Autodesk Inventor part; units mm, degrees
ref_plane "YZ Plane" through (0, 0, 0) normal (1, 0, 0) x (0, 1, 0)
ref_plane "XZ Plane" through (0, 0, 0) normal (0, 1, 0) x (-1, 0, 0)
ref_plane "XY Plane" through (0, 0, 0) normal (0, 0, 1) x (1, 0, 0)
sketch "スケッチ1" plane through (0, 0, 0) normal (0, 0, 1) x (1, 0, 0)
  circle A0 centre (0, 0) radius 1.5
  dimension "d0" = 3
extrude "押し出し1" add sketch "スケッチ1" along normal blind 6
sketch "スケッチ2" plane through (0, 0, 6) normal (0, 0, 1) x (1, 0, 0)
  circle A0 centre (0, 0) radius 1.5
  circle A1 centre (0, 0) radius 3
  dimension "d3" = 6
extrude "押し出し2" add sketch "スケッチ2" along normal blind 2 contours A0 | A1
fillet "フィレット1" radius 2 1 edges at (-3, 0, 8)
thread "ねじ1"
sketch "スケッチ3" plane through (0, 0, 0) normal (0, 0, -1) x (-1, 0, 0)
  circle A0 centre (0, 0) radius 1.5
extrude "押し出し3" add sketch "スケッチ3" along normal blind 2
sketch "スケッチ4" plane through (0, 0, -2) normal (0, 0, -1) x (-1, 0, 0)
  circle A0 centre (0, 0) radius 1.5
extrude "押し出し4" add sketch "スケッチ4" along normal blind 2
sketch "スケッチ5" plane through (0, 0, -4) normal (0, 0, -1) x (-1, 0, 0)
  circle A0 centre (0, 0) radius 1.5
extrude "押し出し5" add sketch "スケッチ5" along normal blind 2
properties part number "SB　12mmなべネジ" material "Steel, Mild"
For this review, take the finished solid that the model builds, in its own axes (mm). A direction names the side the tool comes from. Coordinates: 2 decimals unless noted, no trailing zeros. Loops run counter-clockwise (first coordinate to the right, second up) from the corner with the lowest first, then second, coordinate; pieces in that order, holes last. Notation, with made-up numbers: (32, -6) - (46, -6) arc R32 cw to (46, 27) - close; hole circle Ø5 at (-5, -35.5). An arc over 180 degrees is marked (long way). Return JSON: item names as keys, results as strings.
Item 1: For faces 1 (the flat face through (1.3, -1.3, 6)), 2 (the flat face through (0, 0, 8)), list the 3-axis set-ups (+Z, -Z, +X, -X, +Y, -Y) from which the entire face can be reached by the end or side of a thin tool; tool diameter is ignored.
Determined:
{"face 1": "-Z", "face 2": "+Z, +X, -X, +Y, -Y"}
Item 2: Insertion check: pin 1 (3 mm diameter, centred on x = 1, z = 3.5, fed in from +Y); pin 2 (2 mm diameter, centred on x = -1, z = 1, fed in from -Y). Each pin has a flat end and moves straight along its axis. Give the tip position at first contact, or say it passes through.
Determined:
{"pin 1": "stops at y = 1.5", "pin 2": "stops at y = -1.5"}
Item 3: For line 1 (Z direction, x = 2.75, y = 0.5); line 2 (Y direction, x = -0.5, z = 3.5); line 3 (Z direction, x = -0.75, y = 2.75), list the stretches that pass through material, from the lowest coordinate up.
Determined:
{"line 1": "z = 6 to 6.88", "line 2": "y = -1.41 to 1.41", "line 3": "z = 6 to 6.76"}
Item 4: Take a section at A-A (z = 4). Give the boundary of the cut face in (x, y), then the cut area to 3 significant figures.
Determined:
{"outline": "circle Ø3 at (0, 0)", "area": "7.07 mm2"}
